Source: CAD feature listing. Evaluate the final solid. Frame: model axes, mm. A direction names the side the tool comes from. Coordinates: 2 decimals unless noted, no trailing zeros. Write each loop counter-clockwise with the first axis right and the second up, starting at its lowest first coordinate (ties: lowest second). Pieces come first, ordered by that corner, then holes. Notation, with made-up numbers: (-25.75, 86) - (-13.75, 86) arc R6 cw to (-13.75, 92) - close; hole circle Ø2 at (73.25, 59.25). An arc over 180 degrees is marked (long way). One line per item, written item: value.
from build123d import *

# Parameters (mm, degrees)
BOSS_EXTRUDE1_DEPTH = 38.1
SKETCH2_R           = 9.525
CUT_EXTRUDE1_DEPTH  = 39.1
SKETCH3_W           = 88.9
SKETCH3_H           = 25.4
CUT_EXTRUDE2_DEPTH  = 38.1


with BuildPart() as part:
    # Sketch1 → Boss-Extrude1 (new body)
    with BuildSketch(Plane.XY):
        Polygon((0, 0), (95.25, 0), (81.186706555, 24.358338769), (38.1, 44.45), (19.05, 44.45), (19.05, 31.75), (0, 31.75), align=None)
    extrude(amount=-BOSS_EXTRUDE1_DEPTH)

    # Sketch2 → Cut-Extrude1 (cut, through all)
    with BuildSketch(Plane.XY):
        with Locations((38.1, 19.05)):
            Circle(SKETCH2_R)
    extrude(amount=-CUT_EXTRUDE1_DEPTH, mode=Mode.SUBTRACT)

    # Sketch3 → Cut-Extrude2 (cut)
    with BuildSketch(Plane(origin=(0, 44.45, 0), x_dir=(1, 0, 0), z_dir=(0, 1, 0))):
        with Locations((50.8, 19.05)):
            Rectangle(SKETCH3_W, SKETCH3_H)
    extrude(amount=-CUT_EXTRUDE2_DEPTH, mode=Mode.SUBTRACT)


solid = part.part
1) Reachability of faces 5 (the flat face through (48, 21, -31.75)), 6 (the flat face through (29, 44.45, -35)), 7 (the flat face through (5, 31.75, -19)) from +Z, -Z, +X, -X, +Y, -Y: full face, straight path, thin tool, end or side. Return the list, or none.
Values found:
face 5: +X, +Y
face 6: +Z, -Z, +X, -X, +Y
face 7: +Z, -Z, -X, +Y
2) Section query D-D on z = -18. Output: boundary loops of the cut face in (x, y), then the cut area to 3 significant figures.
Values found:
outline: (0, 0) - (95.25, 0) - (91.58, 6.35) - (6.35, 6.35) - (6.35, 31.75) - (0, 31.75) - close
area: 754 mm2
3) Section query B-B on y = 41.5. Output: boundary loops of the cut face in (x, z).
Values found:
outline: (19.05, -38.1) - (44.43, -38.1) - (44.43, -31.75) - (19.05, -31.75) - close; (19.05, -6.35) - (44.43, -6.35) - (44.43, 0) - (19.05, 0) - close
4) Contact query for flat-ended pins moving along their axis: P1, Ø3, axis at y = 23, z = -9, coming from the +X side; P2, Ø1, axis at x = 79, y = 26.5, coming from the +Z side; P3, Ø9.5, axis at x = 6.5, z = -11, coming from the +Y side; P4, Ø3, axis at y = 35.5, z = -36.5, coming from the -X side. Output: stop coordinate, or through.
Values found:
P1: x = 6.35
P2: through
P3: y = 31.75
P4: x = 19.05
5) Section query A-A on y = 27.5. Output: boundary loops of the cut face in (x, z), then the cut area to 3 significant figures.
Values found:
outline: (0, -38.1) - (33.7, -38.1) - (33.7, -31.75) - (6.35, -31.75) - (6.35, -6.35) - (33.7, -6.35) - (33.7, 0) - (0, 0) - close; (42.5, -38.1) - (74.45, -38.1) - (74.45, -31.75) - (42.5, -31.75) - close; (42.5, -6.35) - (74.45, -6.35) - (74.45, 0) - (42.5, 0) - close
area: 995 mm2
6) Material intervals for line 1 (Z direction, x = 12.5, y = 28.5); line 2 (Y direction, x = 38.1, z = -3.25) (3 decimals); line 3 (Y direction, x = 61.5, z = -9), sorted ascending.
Values found:
line 1: -38.1 to -31.75, -6.35 to 0
line 2: 0 to 9.525, 28.575 to 44.45
line 3: 0 to 6.35
7) Section query C-C on x = 82.5. Output: boundary loops of the cut face in (y, z).
Values found:
outline: (0, -38.1) - (22.08, -38.1) - (22.08, -31.75) - (6.35, -31.75) - (6.35, -6.35) - (22.08, -6.35) - (22.08, 0) - (0, 0) - close
8) Draft query along X for faces 1 (the flat face through (0, 16, -19)), 2 (the cylindrical face through (30.541, 13.254, -34.881)), 3 (the cylindrical face through (30.541, 13.254, -3.131)), 4 (the flat face through (48, 6.35, -19)). Return one class per face: released by +X, released by -X, zero draft, split by the parting line, or undercut.
Values found:
face 1: released by -X
face 2: undercut
face 3: undercut
face 4: zero draft
